Design review of the part shown in the three views and the two pictorial views. Dimensions are in mm from the part's minimum x, y and z. Coordinates: 2 decimals unless noted, no trailing zeros. Loops run counter-clockwise (first coordinate to the right, second up) from the corner with the lowest first, then second, coordinate; pieces in that order, holes last. Notation, with made-up numbers: (-20.75, -16) - (4.25, -16) arc R29 ccw to (4.25, 13) - close; hole circle Ø6 at (-31.5, -34.5). An arc over 180 degrees is marked (long way). One line per item, written item: value. Start each with the question number.
1. Insertion check: pin 1 (1.5 mm diameter, centred on x = 143, y = 59.5, fed in from -Z); pin 2 (1.5 mm diameter, centred on x = 166.5, z = 1, fed in from -Y); pin 3 (1.5 mm diameter, centred on x = 88.5, z = 1, fed in from +Y); pin 4 (1.5 mm diameter, centred on y = 55, z = 1, fed in from -X). Each pin has a flat end and moves straight along its axis. Give the tip position at first contact, or say it passes through.
2. Take a section at B-B, the plane y = 21. State the section outline as (x, z) points, and give its area (3 significant figures).
3. Take a section at C-C, the plane x = 163. State the section outline as (y, z) points, and give its area (3 significant figures).
4. To check wall thickness, follow line 1 (X direction, y = 60.5, z = 0.25); line 2 (Y direction, x = 8, z = 0.65). State the ranges of each line that lie inside material, in increasing order. Write a range as from..to.
5. Take a section at A-A, the plane z = 1.2. State the section outline as (x, y) points, and give its area (3 significant figures).
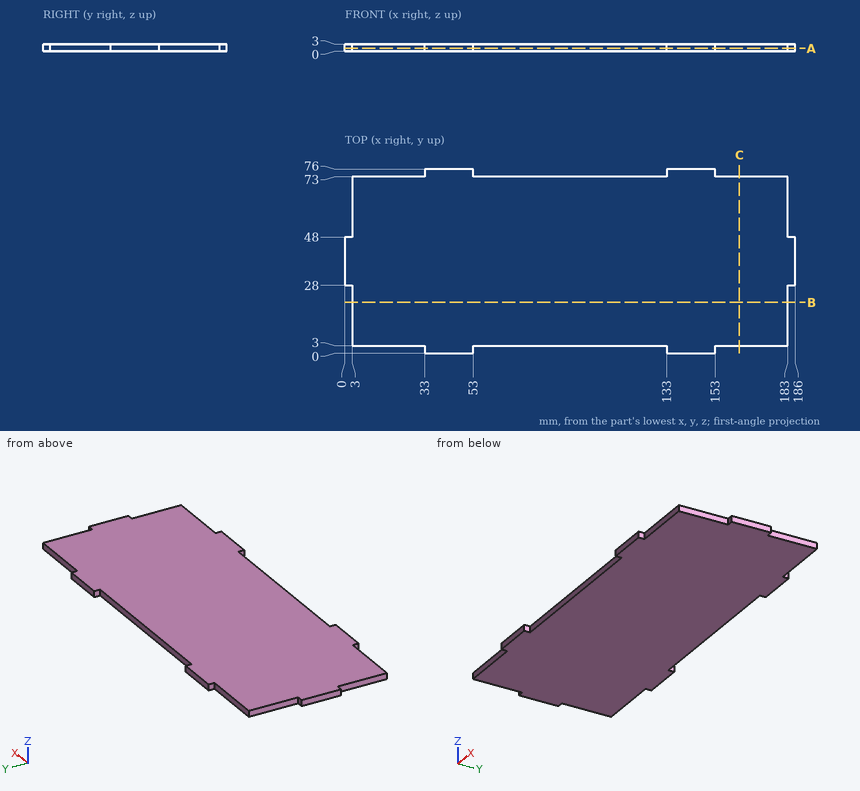
Solutions:
1. pin 1: z = 0
1. pin 2: y = 3
1. pin 3: y = 73
1. pin 4: x = 3
2. outline: (3, 0) - (183, 0) - (183, 3) - (3, 3) - close
2. area: 540 mm2
3. outline: (3, 0) - (73, 0) - (73, 3) - (3, 3) - close
3. area: 210 mm2
4. line 1: 3..183
4. line 2: 3..73
5. outline: (0, 28) - (3, 28) - (3, 3) - (33, 3) - (33, 0) - (53, 0) - (53, 3) - (133, 3) - (133, 0) - (153, 0) - (153, 3) - (183, 3) - (183, 28) - (186, 28) - (186, 48) - (183, 48) - (183, 73) - (153, 73) - (153, 76) - (133, 76) - (133, 73) - (53, 73) - (53, 76) - (33, 76) - (33, 73) - (3, 73) - (3, 48) - (0, 48) - close
5. area: 13,000 mm2
